from build123d import *

# Parameters (mm, degrees)
SKETCH1_R           = 25.5
SKETCH1_R_2         = 20
BOSS_EXTRUDE1_DEPTH = 1
SKETCH1_3_R         = 20
BOSS_EXTRUDE2_DEPTH = 1.8
HOLE1_AT_2_COUNT    = 2
HOLE1_AT_2_PITCH    = 11.313708499
HOLE1_AT_3_COUNT    = 2
HOLE1_AT_3_PITCH    = 16
HOLE1_AT_4_COUNT    = 2
HOLE1_AT_4_PITCH    = 11.313708499


with BuildPart() as part:
    # Sketch1 → Boss-Extrude1 (new body)
    with BuildSketch(Plane.XY):
        Circle(SKETCH1_R)
        Circle(SKETCH1_R_2, mode=Mode.SUBTRACT)
    extrude(amount=BOSS_EXTRUDE1_DEPTH)

    # Sketch1<3> → Boss-Extrude2 (add)
    with BuildSketch(Plane.XY):
        Circle(SKETCH1_3_R)
    extrude(amount=BOSS_EXTRUDE2_DEPTH)

    # Sketch4 → Hole1 (revolve, cut)
    with BuildSketch(Plane(origin=(-8, 0, 1.8), x_dir=(0, -1, 0), z_dir=(1, 0, 0))):
        Polygon((0, 0), (0, 1.8), (1.6, 1.8), (1.6, 1.448533162), (3.1, 0), align=None)
    hole1 = revolve(axis=Axis((-8, 0, 8.245314094), (0, 0, -1)), mode=Mode.SUBTRACT)

    # Hole1 at 2: Hole1 ×2
    with Locations(*[Vector(0.7071067811865276, 0.7071067811865676, 0) * (i * HOLE1_AT_2_PITCH) for i in range(1, HOLE1_AT_2_COUNT)]):
        add(hole1, mode=Mode.SUBTRACT)

    # Hole1 at 3: Hole1 ×2
    with Locations(*[(i * HOLE1_AT_3_PITCH, 0, 0) for i in range(1, HOLE1_AT_3_COUNT)]):
        add(hole1, mode=Mode.SUBTRACT)

    # Hole1 at 4: Hole1 ×2
    with Locations(*[Vector(0.7071067811865676, -0.7071067811865276, 0) * (i * HOLE1_AT_4_PITCH) for i in range(1, HOLE1_AT_4_COUNT)]):
        add(hole1, mode=Mode.SUBTRACT)


solid = part.part
Geometry: final body of the model. Coordinates: model frame, mm. A direction names the side the tool comes from. Give positions to 0.01 mm unless a question says otherwise; leave off trailing zeros. Loops run counter-clockwise (first coordinate to the right, second up) from the corner with the lowest first, then second, coordinate; pieces in that order, holes last. Notation, with made-up numbers: M 33,82 L 72,82 A12 ccw 72,100 Z; hole C -14.75,-16.5 d5. An arc over 180 degrees is marked long. Put each result on its own line as item: value. Start each with the question number.
1) Cut plane A-A (y = 0). Output: boundary loops of the cut face in (x, z).
2) Contact query for flat-ended pins moving along their axis: pin 1 (5 mm diameter, centred on x = 0, y = -8, fed in from +Z); pin 2 (1.9 mm diameter, centred on x = -8, y = 0, fed in from -Z); pin 3 (3.5 mm diameter, centred on x = 8, y = 0, fed in from +Z). Output: stop coordinate, or through.
3) Pull-direction query (X, two-part tool) for faces 1 (the cylindrical face through (1.56, -7.65, 0.18)), 2 (the flat face through (0, 0, 1.8)), 3 (the cylindrical face through (-5.5, -24.9, 0.5)); classes: pulls with the +X half, pulls with the -X half, needs draft (parallel to the pull), parting line crosses it, or undercut.
4) Access query for faces 4 (the cylindrical face through (-0.07, 9.6, 0.18)), 5 (the cylindrical face through (-4.336, -19.524, 1.394)). Directions: +Z, -Z, +X, -X, +Y, -Y. A direction counts if a zero-diameter tool reaches every point of the face in a straight line with its end or side. Return the directions, or none.
5) Cut plane C-C (x = 8). Output: boundary loops of the cut face in (y, z).
6) Ray query, line 1 along Z through (x, y) = (14, 20.5); line 2 along X through (y, z) = (-2, 1.6); line 3 along Y through (x, z) = (-8, 0.15). Return the intervals inside material, ascending.
Verdict:
1. outline: M -25.5,0 L -9.6,0 L -9.6,0.35 L -11.1,1.8 L -20,1.8 L -20,1 L -25.5,1 Z; M -6.4,0 L 6.4,0 L 6.4,0.35 L 4.9,1.8 L -4.9,1.8 L -6.4,0.35 Z; M 9.6,0 L 25.5,0 L 25.5,1 L 20,1 L 20,1.8 L 11.1,1.8 L 9.6,0.35 Z
2. pin 1: z = 1.22
2. pin 2: through
2. pin 3: z = 0.5
3. face 1: undercut
3. face 2: needs draft
3. face 3: parting line crosses it
4. face 4: +Z, -Z
4. face 5: +Z
5. outline: M -24.21,0 L -1.6,0 L -1.6,0.35 L -3.1,1.8 L -18.33,1.8 L -18.33,1 L -24.21,1 Z; M 1.6,0 L 24.21,0 L 24.21,1 L 18.33,1 L 18.33,1.8 L 3.1,1.8 L 1.6,0.35 Z
6. line 1: 0 to 1
6. line 2: -19.9 to -10.09, -5.91 to 5.91, 10.09 to 19.9
6. line 3: -24.21 to -1.6, 1.6 to 24.21
